Source: CAD feature listing. Evaluate the final solid. Frame: model axes, mm. A direction names the side the tool comes from. Give positions to 0.01 mm unless a question says otherwise; leave off trailing zeros. Write each loop counter-clockwise with the first axis right and the second up, starting at its lowest first coordinate (ties: lowest second). Pieces come first, ordered by that corner, then holes. Notation, with made-up numbers: M 51,66 L 64,66 A32 cw 64,100 Z; hole C 51.25,55.5 d10. An arc over 180 degrees is marked long. Answer as a JSON object with one key per item and string values. Group by question number.
```python
from build123d import *

# Parameters (mm, degrees)
SKETCH1_R           = 12
SKETCH1_R_2         = 2.5
BOSS_EXTRUDE1_DEPTH = 6.35
SKETCH2_R           = 5.675
SKETCH2_R_2         = 2.5
BOSS_EXTRUDE2_DEPTH = 6.35
SKETCH3_R           = 5.675
SKETCH3_R_2         = 1.5875
BOSS_EXTRUDE3_DEPTH = 1.5875


with BuildPart() as part:
    # Sketch1 → Boss-Extrude1 (new body)
    with BuildSketch(Plane.XY):
        Circle(SKETCH1_R)
        Circle(SKETCH1_R_2, mode=Mode.SUBTRACT)
    extrude(amount=BOSS_EXTRUDE1_DEPTH)

    # Sketch2 → Boss-Extrude2 (add)
    with BuildSketch(Plane(origin=(0, 0, 0), x_dir=(-1, 0, 0), z_dir=(0, 0, -1))):
        Circle(SKETCH2_R)
        Circle(SKETCH2_R_2, mode=Mode.SUBTRACT)
    extrude(amount=BOSS_EXTRUDE2_DEPTH)

    # Sketch3 → Boss-Extrude3 (add)
    with BuildSketch(Plane(origin=(0, 0, -6.35), x_dir=(-1, 0, 0), z_dir=(0, 0, -1))):
        Circle(SKETCH3_R)
        Circle(SKETCH3_R_2, mode=Mode.SUBTRACT)
    extrude(amount=-BOSS_EXTRUDE3_DEPTH)


solid = part.part
```
(1) Access query for faces 1 (the flat face through (-2, 0, -4.762)), 2 (the flat face through (-1.2, 1.3, -6.35)), 3 (the cylindrical face through (-5.242, -2.174, -3.131)). Directions: +Z, -Z, +X, -X, +Y, -Y. A direction counts if a zero-diameter tool reaches every point of the face in a straight line with its end or side. Return the directions, or none.
(2) Section D-D, the plane y = -3.25. Return loops of the section in (x, z), plus the area to 3 significant figures.
(3) Contact query for flat-ended pins moving along their axis: pin 1 Ø6 at (x, z) = (8, 2.5) entering from +Y; pin 2 Ø2.5 at (x, y) = (-1, 0.5) entering from +Z; pin 3 Ø1.9 at (x, y) = (0, 0) entering from +Z; pin 4 Ø2 at (y, z) = (9, 0.5) entering from -X. Output: stop coordinate, or through.
(4) Section C-C, the plane z = 4.5. Return loops of the section in (x, y).
(5) Ray query, L1, parallel to Y at x = 0, z = -5.8 (1 decimal); L2, parallel to Y at x = 0, z = 3; L3, parallel to Z at x = -6.75, y = 9.25. Return the intervals inside material, ascending. Write a range as [from, to].
Reported:
{
 "1": {"face 1": "+Z", "face 2": "-Z, +X, -X, +Y, -Y", "face 3": "-Z"},
 "2": {"outline": "M -11.55,0 L -4.65,0 L -4.65,-6.35 L 4.65,-6.35 L 4.65,0 L 11.55,0 L 11.55,6.35 L -11.55,6.35 Z", "area": "206 mm2"},
 "3": {"pin 1": "stops at y = 10.91", "pin 2": "stops at z = -4.76", "pin 3": "passes through", "pin 4": "stops at x = -8.94"},
 "4": {"outline": "C 0,0 d24; hole C 0,0 d5"},
 "5": {"L1": "y = [-5.7, -1.6], [1.6, 5.7]", "L2": "y = [-12, -2.5], [2.5, 12]", "L3": "z = [0, 6.35]"}
}
